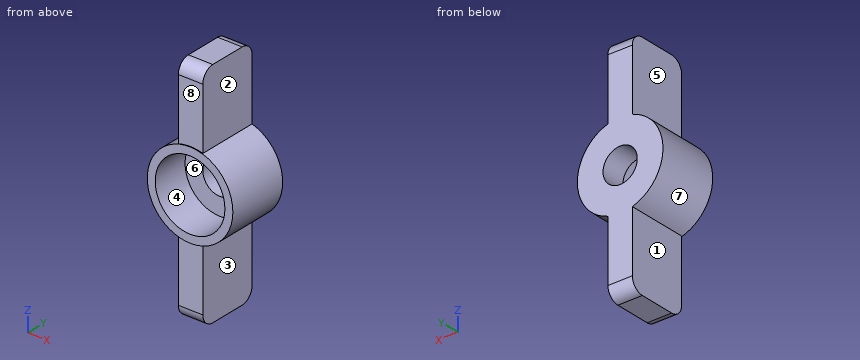
```python
from build123d import *

# Parameters (mm, degrees)
F0_R     = 3.5
F0_R_2   = 1.4
F1_DEPTH = 5
F4_DEPTH = 1
F2_R     = 2.85
F5_DEPTH = 3
F6_R     = 1


with BuildPart() as f1:
    # F0 (on Front) → F1 (new body)
    with BuildSketch(Plane.XZ):
        Circle(F0_R)
        Circle(F0_R_2, mode=Mode.SUBTRACT)
    extrude(amount=F1_DEPTH)

    # F3 (on Right) → F4 (join, symmetric)
    with BuildSketch(Plane.YZ):
        Polygon((0, -3.5), (0, -1.75), (-4.945105, -1.75), (-4.945105, -3.382278), (-4.945105, -3.5), (-4.945105, -9.382278), (0, -9.382278), align=None)
        Polygon((-4.945105, 1.75), (0, 1.75), (0, 3.5), (0, 9.382278), (-4.945105, 9.382278), (-4.945105, 3.5), (-4.945105, 3.382278), align=None)
    extrude(amount=F4_DEPTH, both=True)

    # F2 (on face) → F5 (cut)
    with BuildSketch(Plane.XZ.offset(5)):
        Circle(F2_R)
    extrude(amount=-F5_DEPTH, mode=Mode.SUBTRACT)

    # F6
    f6_edges = [f1.edges().sort_by_distance(p)[0] for p in [
        (0, -4.945105, 9.382278),
        (0, 0, 9.382278),
        (0, -4.945105, -9.382278),
        (0, 0, -9.382278),
    ]]
    fillet(f6_edges, radius=F6_R)


solid = f1.part
```
The model under review builds one solid part; all positions refer to its coordinate system, in mm. Face numbers are marked on the shaded views. A direction names the side the tool comes from. Round coordinates to 2 decimals unless told otherwise and drop trailing zeros. Loops run counter-clockwise (first coordinate to the right, second up) from the corner with the lowest first, then second, coordinate; pieces in that order, holes last.
Item 1: Mouldability with a two-part tool opening along X and no side actions: class the marked faces 5, 6, 7 and 8 as released by +X, released by -X, zero draft, split by the parting line, or undercut.
Determined:
face 5: released by -X
face 6: undercut
face 7: split by the parting line
face 8: zero draft
Item 2: Take a section at C-C (y = -2.2). Write out the cut boundary in (x, z), then the cut area to 3 significant figures.
Determined:
outline: (-1, -9.38) - (1, -9.38) - (1, -3.35) arc R3.5 ccw to (1, 3.35) - (1, 9.38) - (-1, 9.38) - (-1, 3.35) arc R3.5 ccw to (-1, -3.35) - close; hole circle Ø5.7 at (0, 0)
area: 36.7 mm2
Item 3: Take a section at B-B (x = 0). Write out the cut boundary in (y, z), then the cut area to 3 significant figures.
Determined:
outline: (-5, -3.5) - (-4.95, -3.5) - (-4.95, -8.38) arc R1 ccw to (-3.95, -9.38) - (-1, -9.38) arc R1 ccw to (0, -8.38) - (0, -1.4) - (-2, -1.4) - (-2, -2.85) - (-5, -2.85) - close; (-5, 2.85) - (-2, 2.85) - (-2, 1.4) - (0, 1.4) - (0, 8.38) arc R1 ccw to (-1, 9.38) - (-3.95, 9.38) arc R1 ccw to (-4.95, 8.38) - (-4.95, 3.5) - (-5, 3.5) - close
area: 69.6 mm2
Item 4: Clearance check with flat-ended pins moving along their axes: pin 1 Ø2.5 at (y, z) = (-3.5, 5) entering from +X; pin 2 Ø1 at (y, z) = (-1.5, -4.5) entering from -X; pin 3 Ø0.6 at (x, z) = (-0.5, 5.5) entering from -Y. State where each tip first meets the part, or that it passes through.
Determined:
pin 1: stops at x = 1
pin 2: stops at x = -1
pin 3: stops at y = -4.95
Item 5: Take a section at D-D (x = 2.5). Write out the cut boundary in (y, z).
Determined:
outline: (-5, -2.45) - (0, -2.45) - (0, 2.45) - (-5, 2.45) - (-5, 1.37) - (-2, 1.37) - (-2, -1.37) - (-5, -1.37) - close
Item 6: For the marked faces 1, 2, 3 and 4, list the 3-axis set-ups (+Z, -Z, +X, -X, +Y, -Y) from which the entire face can be reached by the end or side of a thin tool; tool diameter is ignored.
Determined:
face 1: -Z, -X, +Y, -Y
face 2: +Z, +X, +Y, -Y
face 3: -Z, +X, +Y, -Y
face 4: -Y
Item 7: Take a section at A-A (z = 0). Write out the cut boundary in (x, y).
Determined:
outline: (-3.5, -5) - (-2.85, -5) - (-2.85, -2) - (-1.4, -2) - (-1.4, 0) - (-3.5, 0) - close; (1.4, -2) - (2.85, -2) - (2.85, -5) - (3.5, -5) - (3.5, 0) - (1.4, 0) - close
Item 8: For line 1 (Z direction, x = 0, y = -3.2); line 2 (Z direction, x = 0, y = -1.1); line 3 (X direction, y = -3.4, z = -8.25), list the stretches that pass through material, from the lowest coordinate up.
Determined:
line 1: z = -9.38 to -2.85, 2.85 to 9.38
line 2: z = -9.38 to -1.4, 1.4 to 9.38
line 3: x = -1 to 1
